Could you check a few things on this model? Use its own coordinates, in mm. A direction names the side the tool comes from. Coordinates: 2 decimals unless noted, no trailing zeros. Order: outer loops, then holes, each group sorted by start corner. A loop starts at its lowest first (then second) coordinate and runs counter-clockwise, first axis right, second up. Notation, with made-up numbers: (62, 2) - (85, 2) arc R34 cw to (85, 40) - close; hole circle Ø3 at (85.25, 80). An arc over 180 degrees is marked (long way). Answer as a JSON object with one key per item and string values. Group by question number.
(1) Imagine slicing it at A-A, the plane y = -6.75. Write out the boundary of the cut face in (x, z), and give its area (3 significant figures).
(2) Please list where these lines run through material, in increasing order: probe 1 along X at (y, z) = (-9, 3); probe 2 along Y at (x, z) = (-8.5, 26).
(3) Imagine slicing it at C-C, the plane x = -11. Write out the boundary of the cut face in (y, z).
(4) Imagine slicing it at B-B, the plane z = 49. Write out the boundary of the cut face in (x, y), and give its area (3 significant figures).
(5) Imagine slicing it at D-D, the plane y = -4. Write out the boundary of the cut face in (x, z).
(6) Which directions (+Z, -Z, +X, -X, +Y, -Y) give clear straight access to the entire face, cutting with the end or side of a thin tool? Please do faces 5 (the flat face through (-10, -3, 30)), 6 (the flat face through (-19.5, -10, 29.6)), 7 (the flat face through (-1, -20, 30)).
(7) We'd pull the mould along X, two halves only. Please class faces 1 (the flat face through (-8.1, -2.5, 0)), 2 (the cylindrical face through (-16, -4, 30)), 3 (the cylindrical face through (-20.699, -9.715, 29.58)), 4 (the flat face through (0, -10, 30)): pulls with the +X half, pulls with the -X half, needs draft (parallel to the pull), parting line crosses it, or undercut.
(8) Will these pins go through, and if not, where does the flat tip stop? P1, Ø1.5, axis at x = -10, z = 45, coming from the -Y side; P2, Ø3, axis at x = -15.5, z = 52, coming from the -Y side; P3, Ø6, axis at y = -13.5, z = 19, coming from the -X side.
from build123d import *

# Parameters (mm, degrees)
BOSS_EXTRUDE1_DEPTH = 60


with BuildPart() as part:
    # Sketch1 → Boss-Extrude1 (new body)
    with BuildSketch(Plane.XY):
        with BuildLine():
            Line((0, 0), (0, -20))
            Line((0, -20), (-3, -20))
            Line((-3, -20), (-3, -8))
            ThreePointArc((-3, -8), (-4.464466094, -4.464466094), (-8, -3))
            Line((-8, -3), (-13, -3))
            ThreePointArc((-13, -3), (-16.535533906, -4.464466094), (-18, -8))
            Line((-18, -8), (-18, -9))
            ThreePointArc((-18, -9), (-18.292893219, -9.707106781), (-19, -10))
            Line((-19, -10), (-20, -10))
            ThreePointArc((-20, -10), (-20.707106781, -9.707106781), (-21, -9))
            Line((-21, -9), (-21, -5))
            ThreePointArc((-21, -5), (-19.535533906, -1.464466094), (-16, 0))
            Line((-16, 0), (0, 0))
        make_face()
    extrude(amount=BOSS_EXTRUDE1_DEPTH)


solid = part.part
Result set:
{
 "1": {"outline": "(-21, 0) - (-17.84, 0) - (-17.84, 60) - (-21, 60) - close; (-3.16, 0) - (0, 0) - (0, 60) - (-3.16, 60) - close", "area": "379 mm^2"},
 "2": {"probe 1": "x = -21 to -18, -3 to 0", "probe 2": "y = -3 to 0"},
 "3": {"outline": "(-3, 0) - (0, 0) - (0, 60) - (-3, 60) - close"},
 "4": {"outline": "(-21, -9) arc R1 ccw to (-20, -10) - (-19, -10) arc R1 ccw to (-18, -9) - (-18, -8) arc R5 cw to (-13, -3) - (-8, -3) arc R5 cw to (-3, -8) - (-3, -20) - (0, -20) - (0, 0) - (-16, 0) arc R5 ccw to (-21, -5) - close", "area": "140 mm^2"},
 "5": {"outline": "(-20.9, 0) - (-16, 0) - (-16, 60) - (-20.9, 60) - close; (-5, 0) - (0, 0) - (0, 60) - (-5, 60) - close"},
 "6": {"face 5": "+Z, -Z, -Y", "face 6": "+Z, -Z, -X, -Y", "face 7": "+Z, -Z, +X, -X, -Y"},
 "7": {"face 1": "needs draft", "face 2": "undercut", "face 3": "pulls with the -X half", "face 4": "pulls with the +X half"},
 "8": {"P1": "stops at y = -3", "P2": "stops at y = -5", "P3": "stops at x = -3"}
}
